Design review of the part built by this model. Coordinates are the model's own, in mm. Face numbers are marked on the shaded views. A direction names the side the tool comes from. Coordinates: 2 decimals unless noted, no trailing zeros. Order: outer loops, then holes, each group sorted by start corner. A loop starts at its lowest first (then second) coordinate and runs counter-clockwise, first axis right, second up. Notation, with made-up numbers: M -18,-11.5 L 3,-11.5 A24 cw 3,6.5 Z; hole C 55.5,39 d9. An arc over 180 degrees is marked long. Answer in a Markdown table with one row per item.
from build123d import *

# Parameters (mm, degrees)
SKETCH_1_W          = 26
SKETCH_1_H          = 38
EXTRUDE_1_DEPTH     = 10
SKETCH_2_W          = 22
SKETCH_2_H          = 34
CUT_EXTRUDE_1_DEPTH = 8
SKETCH_4_W          = 6
SKETCH_4_H          = 6
EXTRUDE_2_DEPTH     = 2
SKETCH_5_R          = 1
CUT_EXTRUDE_4_DEPTH = 2
FILLET_1_R          = 5


with BuildPart() as part:
    # ｽｹｯﾁ1 → ﾎﾞｽ - 押し出し1 (new body)
    with BuildSketch(Plane.XY):
        Rectangle(SKETCH_1_W, SKETCH_1_H)
    extrude(amount=EXTRUDE_1_DEPTH)

    # ｽｹｯﾁ2 → ｶｯﾄ - 押し出し1 (cut)
    with BuildSketch(Plane.XY):
        Rectangle(SKETCH_2_W, SKETCH_2_H)
    extrude(amount=CUT_EXTRUDE_1_DEPTH, mode=Mode.SUBTRACT)

    # ｽｹｯﾁ4 → ﾎﾞｽ - 押し出し2 (add)
    with BuildSketch(Plane.XY):
        with Locations((16, 16)):
            Rectangle(SKETCH_4_W, SKETCH_4_H)
        with Locations((16, -16)):
            Rectangle(SKETCH_4_W, SKETCH_4_H)
        with Locations((-16, -16)):
            Rectangle(SKETCH_4_W, SKETCH_4_H)
        with Locations((-16, 16)):
            Rectangle(SKETCH_4_W, SKETCH_4_H)
    extrude(amount=EXTRUDE_2_DEPTH)

    # ｽｹｯﾁ5 → ｶｯﾄ - 押し出し4 (cut)
    with BuildSketch(Plane.XY):
        with Locations((-16, 16)):
            Circle(SKETCH_5_R)
        with Locations((-16, -16)):
            Circle(SKETCH_5_R)
        with Locations((16, -16)):
            Circle(SKETCH_5_R)
        with Locations((16, 16)):
            Circle(SKETCH_5_R)
    extrude(amount=CUT_EXTRUDE_4_DEPTH, mode=Mode.SUBTRACT)

    # ﾌｨﾚｯﾄ1
    fillet_1_edges = [part.edges().sort_by_distance(p)[0] for p in [
        (0, 19, 10),
        (0, -19, 10),
        (13, 0, 10),
        (-13, 0, 10),
    ]]
    fillet(fillet_1_edges, radius=FILLET_1_R)


solid = part.part
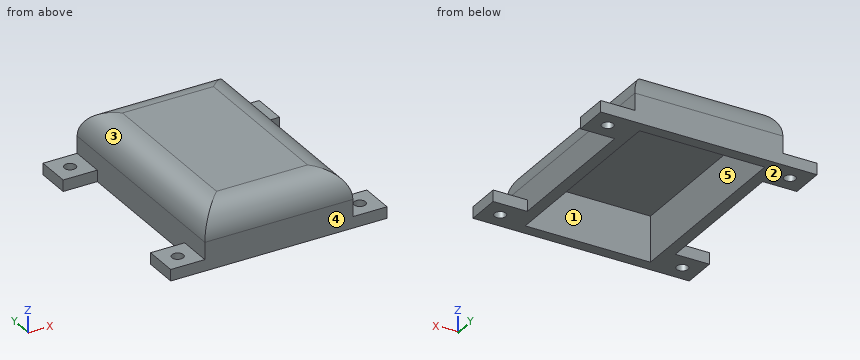
(1) Add section C-C, the plane z = 1.5. Give the boundary of the cut face in (x, y), and give its area (3 significant figures).
Return value:
| item | result |
|---|---|
| outline | M -19,-19 L 19,-19 L 19,-13 L 13,-13 L 13,13 L 19,13 L 19,19 L -19,19 L -19,13 L -13,13 L -13,-13 L -19,-13 Z; hole C -16,-16 d2; hole C -16,16 d2; hole M -11,-17 L 11,-17 L 11,17 L -11,17 Z; hole C 16,-16 d2; hole C 16,16 d2 |
| area | 371 mm2 |
(2) Draft analysis for pull direction X (two halves, no side actions). For the marked faces 3, 4 and 5, state which applies: pulls with the +X half, pulls with the -X half, needs draft (parallel to the pull), parting line crosses it, or undercut.
Return value:
| item | result |
|---|---|
| face 3 | pulls with the -X half |
| face 4 | needs draft |
| face 5 | undercut |
(3) Add section A-A, the plane x = -16. Give the boundary of the cut face in (y, z).
Return value:
| item | result |
|---|---|
| outline | M -19,0 L -17,0 L -17,2 L -19,2 Z; M -15,0 L -13,0 L -13,2 L -15,2 Z; M 13,0 L 15,0 L 15,2 L 13,2 Z; M 17,0 L 19,0 L 19,2 L 17,2 Z |
(4) Add section B-B, the plane z = 3.5. Give the boundary of the cut face in (x, y).
Return value:
| item | result |
|---|---|
| outline | M -13,-19 L 13,-19 L 13,19 L -13,19 Z; hole M -11,-17 L 11,-17 L 11,17 L -11,17 Z |
(5) For the marked faces 1 and 2, list the 3-axis set-ups (+Z, -Z, +X, -X, +Y, -Y) from which the entire face can be reached by the end or side of a thin tool; tool diameter is ignored.
Return value:
| item | result |
|---|---|
| face 1 | -Z |
| face 2 | -Z, +X, -X, +Y, -Y |
(6) Insertion check: pin 1 Ø4 at (y, z) = (9, 4.5) entering from -X; pin 2 Ø8 at (x, y) = (14, -7.5) entering from -Z; pin 3 Ø1.5 at (y, z) = (3.5, 2) entering from +X; pin 4 Ø2.5 at (x, y) = (16, 16) entering from +Z. Each pin has a flat end and moves straight along its axis. Give the tip position at first contact, or say it passes through.
Return value:
| item | result |
|---|---|
| pin 1 | stops at x = -13 |
| pin 2 | stops at z = 0 |
| pin 3 | stops at x = 13 |
| pin 4 | stops at z = 2 |
(7) For line 1 along Y through (x, z) = (16, 0.9); line 2 along Y through (x, z) = (2.5, 5.25); line 3 along X through (y, z) = (4.5, 4), list the stretches that pass through material, from the lowest coordinate up. Write a range as from..to.
Return value:
| item | result |
|---|---|
| line 1 | y = -19..-17, -15..-13, 13..15, 17..19 |
| line 2 | y = -18.99..-17, 17..18.99 |
| line 3 | x = -13..-11, 11..13 |
(8) Add section D-D, the plane y = -15.5. Give the boundary of the cut face in (x, z).
Return value:
| item | result |
|---|---|
| outline | M -19,0 L -16.87,0 L -16.87,2 L -19,2 Z; M -15.13,0 L -11,0 L -11,8 L 11,8 L 11,0 L 15.13,0 L 15.13,2 L 13,2 L 13,5 A5 ccw 9.5,9.77 L -9.5,9.77 A5 ccw -13,5 L -13,2 L -15.13,2 Z; M 16.87,0 L 19,0 L 19,2 L 16.87,2 Z |
